Work out the finished part from the listing and answer in its coordinate system (mm). A direction names the side the tool comes from. Coordinates: 2 decimals unless noted, no trailing zeros. Write each loop counter-clockwise with the first axis right and the second up, starting at its lowest first coordinate (ties: lowest second). Pieces come first, ordered by that corner, then holes. Notation, with made-up numbers: (85, 38) - (103, 38) arc R10 ccw to (103, 44) - close; hole circle Ø7 at (6, 66.5). An arc over 180 degrees is marked (long way). Use a Markdown table: item, result. Add a question column.
(1) Given pin 1 Ø6 at (x, y) = (541.5, -570) entering from -Z; pin 2 Ø1.5 at (x, z) = (255, -297) entering from +Y; pin 3 Ø10 at (y, z) = (-498, -189.5) entering from +X, each flat-ended and moving along its own axis, determine where each tip first touches the part or whether it passes through.
(2) A tool of negligible diameter and unlimited length cuts with its end or side. For faces 1 (the face through (1485, -685.8, -502)), 2 (the face through (76.2, -38, -502)), 3 (the face through (38, -76.2, -502)), 4 (the face through (38, -685.8, -502)), 5 (the face through (1447.8, -38, -502)), from which of +Z, -Z, +X, -X, +Y, -Y can it reach the whole face along a straight path? Write none if from no direction.
(3) The part is cut by section A-A, the plane z = -605.5. Give the vertices of the cut face in (x, y).
(4) The part is cut by section C-C, the plane x = 317. Give the vertices of the cut face in (y, z).
(5) For a pull along X with two mould halves and no side action, classify faces 6 (the face through (533.4, -612, -205)), 7 (the face through (1485, -76.2, -502)), 8 (the face through (751, -376, -50.8)), 9 (the face through (0, -69, -409)) as released by +X, released by -X, zero draft, split by the parting line, or undercut.
(6) The part is cut by section D-D, the plane z = -118. Give the vertices of the cut face in (x, y).
(7) Find the intervals of material crossed by line 1 (X direction, y = -57, z = -875); line 2 (Z direction, x = 367, y = -491.5); line 3 (Z direction, x = 840.5, y = -491), in increasing order. Write a range as from..to.
(8) The part is cut by section B-B, the plane y = -555.5. Give the vertices of the cut face in (x, z).
from build123d import *

# Parameters (mm, degrees)
F0_W     = 1524
F0_H     = 762
F1_DEPTH = 50.8
F2_W     = 76.2
F2_H     = 76.2
F3_DEPTH = 914.4
F4_W     = 457.2
F4_H     = 304.8
F5_DEPTH = 304.8


with BuildPart() as f1:
    # F0 (on Top) → F1 (new body)
    with BuildSketch(Plane.XY):
        with Locations((762, -381)):
            Rectangle(F0_W, F0_H)
    extrude(amount=-F1_DEPTH)

    # F2 (on face) → F3 (join)
    with BuildSketch(Plane(origin=(0, 0, -50.8), x_dir=(1, 0, 0), z_dir=(0, 0, -1))):
        with Locations((38.1, 723.9)):
            Rectangle(F2_W, F2_H)
        with Locations((38.1, 38.1)):
            Rectangle(F2_W, F2_H)
        with Locations((1485.9, 38.1)):
            Rectangle(F2_W, F2_H)
        with Locations((1485.9, 723.9)):
            Rectangle(F2_W, F2_H)
    extrude(amount=F3_DEPTH)

    # F4 (on face) → F5 (join)
    with BuildSketch(Plane.XZ.offset(762)):
        with Locations((304.8, -203.2)):
            Rectangle(F4_W, F4_H)
    extrude(amount=-F5_DEPTH)


solid = f1.part
Model answer:
| question | item | result |
|---|---|---|
| 1 | pin 1 | z = -50.8 |
| 1 | pin 2 | y = -457.2 |
| 1 | pin 3 | x = 533.4 |
| 2 | face 1 | -Z, +X |
| 2 | face 2 | -Z, +Y |
| 2 | face 3 | -Z, +X, -X |
| 2 | face 4 | -Z, -X |
| 2 | face 5 | -Z, +Y, -Y |
| 3 | outline | (0, -762) - (76.2, -762) - (76.2, -685.8) - (0, -685.8) - close; (0, -76.2) - (76.2, -76.2) - (76.2, 0) - (0, 0) - close; (1447.8, -762) - (1524, -762) - (1524, -685.8) - (1447.8, -685.8) - close; (1447.8, -76.2) - (1524, -76.2) - (1524, 0) - (1447.8, 0) - close |
| 4 | outline | (-762, -355.6) - (-457.2, -355.6) - (-457.2, -50.8) - (0, -50.8) - (0, 0) - (-762, 0) - close |
| 5 | face 6 | undercut |
| 5 | face 7 | zero draft |
| 5 | face 8 | undercut |
| 5 | face 9 | released by -X |
| 6 | outline | (0, -762) - (533.4, -762) - (533.4, -457.2) - (76.2, -457.2) - (76.2, -685.8) - (0, -685.8) - close; (0, -76.2) - (76.2, -76.2) - (76.2, 0) - (0, 0) - close; (1447.8, -762) - (1524, -762) - (1524, -685.8) - (1447.8, -685.8) - close; (1447.8, -76.2) - (1524, -76.2) - (1524, 0) - (1447.8, 0) - close |
| 7 | line 1 | 0..76.2, 1447.8..1524 |
| 7 | line 2 | -355.6..0 |
| 7 | line 3 | -50.8..0 |
| 8 | outline | (0, -50.8) - (76.2, -50.8) - (76.2, -355.6) - (533.4, -355.6) - (533.4, -50.8) - (1524, -50.8) - (1524, 0) - (0, 0) - close |
